from build123d import *

# Parameters (mm, degrees)
SKETCH001_R  = 5
POCKET_DEPTH = 2.7


with BuildPart() as part:
    # Sketch → Revolution (revolve)
    with BuildSketch(Plane.XZ):
        Polygon((2.5, 0), (2.1, 0.23094), (2.1, 2.46906), (2.5, 2.7), (5, 2.7), (5, 0), align=None)
    revolve(axis=Axis((0, 0, 0), (0, 0, 1)))

    # Sketch001 → Pocket (cut)
    with BuildSketch(Plane(origin=(0, 0, 2.7), x_dir=(-1, 0, 0), z_dir=(0, 0, 1))):
        Circle(SKETCH001_R)
        Polygon((-4, 2.309401), (-4, -2.309401), (0, -4.618802), (4, -2.309401), (4, 2.309401), (0, 4.618802), align=None, mode=Mode.SUBTRACT)
    extrude(amount=-POCKET_DEPTH, mode=Mode.SUBTRACT)


solid = part.part
Verification items for the finished model (mm, model axes). Give positions to 0.01 mm unless a question says otherwise; leave off trailing zeros. Write each loop counter-clockwise with the first axis right and the second up, starting at its lowest first coordinate (ties: lowest second). Pieces come first, ordered by that corner, then holes.
(1) Cross-section at A-A (y = 0). Enter the section's corners in (x, z), plus the area to 3 significant figures.
(2) Mould release check, pull along Y, two halves, no side actions. Record for faces 1 (the face through (2.003, 0.631, 1.366)), 2 (the face through (-1.97, 3.48, 1.37)), 3 (the face through (1.97, -3.48, 1.37)), 4 (the face through (-4, 0, 1)): +Y half, -Y half, draft (parallel to the pull), parting line (faces both ways), or undercut.
(3) Gauge pin test, flat ends, axial feed: pin 1 (1.5 mm diameter, centred on y = -3, z = 0.5, fed in from +X); pin 2 (1.5 mm diameter, centred on x = 2.5, z = 1.5, fed in from -Y); pin 3 (2 mm diameter, centred on x = 1, y = -1, fed in from -Z); pin 4 (1.5 mm diameter, centred on x = -1.5, z = 0.5, fed in from -Y). Record the tip position at first contact, or that the pin passes through.
(4) Cross-section at B-B (z = 0.7). Enter the section's corners in (x, y), plus the area to 3 significant figures.
(5) Material ranges on line 1 (Y direction, x = -0.25, z = 1.25); line 2 (Y direction, x = 1.5, z = 0.55); line 3 (X direction, y = 0.25, z = 2.2), recorded low to high.
Worked out:
1. outline: (-4, 0) - (-2.5, 0) - (-2.1, 0.23) - (-2.1, 2.47) - (-2.5, 2.7) - (-4, 2.7) - close; (2.1, 0.23) - (2.5, 0) - (4, 0) - (4, 2.7) - (2.5, 2.7) - (2.1, 2.47) - close
1. area: 10.1 mm2
2. face 1: undercut
2. face 2: +Y half
2. face 3: -Y half
2. face 4: draft
3. pin 1: stops at x = 4
3. pin 2: stops at y = -3.61
3. pin 3: stops at z = 0.05
3. pin 4: stops at y = -4.19
4. outline: (-4, -2.31) - (0, -4.62) - (4, -2.31) - (4, 2.31) - (0, 4.62) - (-4, 2.31) - close; hole circle Ø4.2 at (0, 0)
4. area: 41.6 mm2
5. line 1: y = -4.47 to -2.09, 2.09 to 4.47
5. line 2: y = -3.75 to -1.47, 1.47 to 3.75
5. line 3: x = -4 to -2.09, 2.09 to 4
